Geometry: final body of the model. Coordinates: model frame, mm. Coordinates: 2 decimals unless noted, no trailing zeros. Loops run counter-clockwise (first coordinate to the right, second up) from the corner with the lowest first, then second, coordinate; pieces in that order, holes last. Notation, with made-up numbers: (-20, 84) -> (34, 84) arc R20 cw to (34, 96) -> close; hole circle Ø5 at (73, 43.25). An arc over 180 degrees is marked (long way). One line per item, written item: value. Start each with the question number.
Item 1: Section query A-A on x = 0.6. Return loops of the section in (y, z).
Item 2: Mould query, pull axis Y, two halves, no side actions, for faces 1 (the cylindrical face through (1.25, 235.97, -190.85)), 2 (the flat face through (2.54, 188, -194)), 3 (the flat face through (1.252, 275.428, -183.467)). Classes: +Y half, -Y half, draft (parallel to the pull), parting line (faces both ways), or undercut.
Item 3: Section query B-B on y = 271. Return loops of the section in (x, z), then the cut area to 3 significant figures.
Item 4: Contact query for flat-ended pins moving along their axis: pin 1 Ø14.5 at (y, z) = (206.36, -193.55) entering from +X; pin 2 Ø1 at (x, y) = (1, 309.5) entering from +Z. Output: stop coordinate, or through.
Item 5: Ray query, probe 1 along Y at (x, z) = (1.8, -201); probe 2 along Z at (x, y) = (1.65, 286.5); probe 3 along Z at (x, y) = (0.45, 178). Return the intervals inside material, ascending. Write a range as from..to.
from build123d import *

# Parameters (mm, degrees)
SKETCH1_R           = 9.7234375
SKETCH1_R_2         = 15.24
SKETCH1_R_3         = 6.35
BOSS_EXTRUDE1_DEPTH = 2.54


with BuildPart() as part:
    # Sketch1 → Boss-Extrude1 (new body)
    with BuildSketch(Plane(origin=(0, 0, 0), x_dir=(0, 0, -1), z_dir=(1, 0, 0))):
        Polygon((199.119533938, 358.909346267), (167.369533938, 189.576012933), (167.369533938, 76.016846267), (211.819533938, 76.016846267), (211.819533938, 308.109346267), (211.819533938, 358.909346267), align=None)
        with Locations((189.594533938, 135.865596267)):
            Circle(SKETCH1_R, mode=Mode.SUBTRACT)
        with Locations((189.594533938, 101.416846267)):
            Circle(SKETCH1_R_2, mode=Mode.SUBTRACT)
        with Locations((191.572880687, 181.032184657)):
            Circle(SKETCH1_R_3, mode=Mode.SUBTRACT)
        with Locations((193.551227437, 206.355023047)):
            Circle(SKETCH1_R_3, mode=Mode.SUBTRACT)
        with Locations((195.529574186, 231.677861438)):
            Circle(SKETCH1_R_3, mode=Mode.SUBTRACT)
        with Locations((197.507920935, 257.000699828)):
            Circle(SKETCH1_R_3, mode=Mode.SUBTRACT)
        with Locations((198.308463246, 282.388081182)):
            Circle(SKETCH1_R_3, mode=Mode.SUBTRACT)
    extrude(amount=BOSS_EXTRUDE1_DEPTH)


solid = part.part
Reply:
1. outline: (76.02, -211.82) -> (358.91, -211.82) -> (358.91, -199.12) -> (189.58, -167.37) -> (76.02, -167.37) -> close; hole circle Ø30.48 at (101.42, -189.59); hole circle Ø19.45 at (135.87, -189.59); hole circle Ø12.7 at (181.03, -191.57); hole circle Ø12.7 at (206.36, -193.55); hole circle Ø12.7 at (231.68, -195.53); hole circle Ø12.7 at (257, -197.51); hole circle Ø12.7 at (282.39, -198.31)
2. face 1: undercut
2. face 2: draft
2. face 3: +Y half
3. outline: (0, -211.82) -> (2.54, -211.82) -> (2.54, -182.64) -> (0, -182.64) -> close
3. area: 74.1 mm²
4. pin 1: stops at x = 2.54
4. pin 2: stops at z = -189.76
5. probe 1: y = 76.02..91.31, 111.52..228.45, 234.9..251.7, 262.3..276.64, 288.14..358.91
5. probe 2: z = -211.82..-203.15, -193.47..-185.54
5. probe 3: z = -211.82..-197.15, -185.99..-167.37
